from build123d import *

# Parameters (mm, degrees)
BOSS_EXTRUDE1_DEPTH = 6.35
SKETCH2_R           = 1.651
BOSS_EXTRUDE2_DEPTH = 6.35
SKETCH4_W           = 4.445
SKETCH4_H           = 4.445
BOSS_EXTRUDE3_DEPTH = 155.575


with BuildPart() as part:
    # Sketch1 → Boss-Extrude1 (new body)
    with BuildSketch(Plane.XY):
        Polygon((0, 0), (6.35, 0), (0, 14.478), (-6.35, 14.478), align=None)
    extrude(amount=BOSS_EXTRUDE1_DEPTH)

    # Sketch2 → Boss-Extrude2 (add)
    with BuildSketch(Plane.XZ):
        with BuildLine():
            Line((6.35, 18.669), (6.35, -12.319))
            ThreePointArc((6.35, -12.319), (3.175, -15.494), (0, -12.319))
            Line((0, -12.319), (0, 18.669))
            ThreePointArc((0, 18.669), (3.175, 21.844), (6.35, 18.669))
        make_face()
        with Locations((3.175, 18.669)):
            Circle(SKETCH2_R, mode=Mode.SUBTRACT)
        with Locations((3.175, -12.319)):
            Circle(SKETCH2_R, mode=Mode.SUBTRACT)
    extrude(amount=BOSS_EXTRUDE2_DEPTH)

    # Sketch4 → Boss-Extrude3 (add)
    with BuildSketch(Plane(origin=(0, 14.478, 0), x_dir=(1, 0, 0), z_dir=(0, 1, 0))):
        with Locations((-3.175, -3.175)):
            Rectangle(SKETCH4_W, SKETCH4_H)
    extrude(amount=BOSS_EXTRUDE3_DEPTH)


solid = part.part
Work out the finished part from the listing and answer in its coordinate system (mm). A direction names the side the tool comes from. Round coordinates to 2 decimals unless told otherwise and drop trailing zeros. Write each loop counter-clockwise with the first axis right and the second up, starting at its lowest first coordinate (ties: lowest second). Pieces come first, ordered by that corner, then holes. Notation, with made-up numbers: M 22,12 L 79,12 A21 ccw 79,47 Z; hole C 52.5,15 d6. An arc over 180 degrees is marked long. Use a Markdown table: item, result.
1) Consider line 1 (Z direction, x = -2.5, y = 7.5); line 2 (Z direction, x = -4.25, y = 157); line 3 (X direction, y = 74, z = 3). Determine where each line is inside the solid, lowest interval first. Write a range as [from, to].
Taken from the geometry:
| item | result |
|---|---|
| line 1 | z = [0, 6.35] |
| line 2 | z = [0.95, 5.4] |
| line 3 | x = [-5.4, -0.95] |
2) The part is cut by section B-B on y = 133. Give the vertices of the cut face in (x, z).
Taken from the geometry:
| item | result |
|---|---|
| outline | M -5.4,0.95 L -0.95,0.95 L -0.95,5.4 L -5.4,5.4 Z |
3) Flat-ended cylindrical pins translate along their axes: pin 1 (2 mm diameter, centred on x = 0, z = 11, fed in from +Y); pin 2 (5 mm diameter, centred on x = -3.5, y = 130.5, fed in from -Z); pin 3 (5 mm diameter, centred on y = 85, z = 2.5, fed in from +X). Find the tip coordinate at first contact, or state that the pin passes through.
Taken from the geometry:
| item | result |
|---|---|
| pin 1 | stops at y = 0 |
| pin 2 | stops at z = 0.95 |
| pin 3 | stops at x = -0.95 |
4) The part is cut by section C-C on z = -7.5. Give the vertices of the cut face in (x, y), plus the area to 3 significant figures.
Taken from the geometry:
| item | result |
|---|---|
| outline | M 0,-6.35 L 6.35,-6.35 L 6.35,0 L 0,0 Z |
| area | 40.3 mm2 |
5) The part is cut by section A-A on z = 3.5. Give the vertices of the cut face in (x, y).
Taken from the geometry:
| item | result |
|---|---|
| outline | M -6.35,14.48 L 0,0 L 0,-6.35 L 6.35,-6.35 L 6.35,0 L 0,14.48 L -0.95,14.48 L -0.95,170.05 L -5.4,170.05 L -5.4,14.48 Z |
6) Determine the mould class of faces 6 (the face through (3.22, 7.14, 3.13)), 7 (the face through (3.105, -3.131, 21.843)), 8 (the face through (2.96, -3.131, -10.682)), 9 (the face through (2.96, -3.131, 20.306)) for opening direction X: pulls with the +X half, pulls with the -X half, needs draft (parallel to the pull), parting line crosses it, or undercut.
Taken from the geometry:
| item | result |
|---|---|
| face 6 | pulls with the +X half |
| face 7 | parting line crosses it |
| face 8 | undercut |
| face 9 | undercut |
7) Which of the six approach directions +Z, -Z, +X, -X, +Y, -Y give full straight-line access (tool end or side, diameter ignored) to faces 1 (the face through (-3, 91, 5.398)), 2 (the face through (-5.398, 91, 3)), 3 (the face through (-0.952, 91, 3)), 4 (the face through (6.35, -3, 3)), 5 (the face through (-3, 91, 0.952))?
Taken from the geometry:
| item | result |
|---|---|
| face 1 | +Z, +X, -X, +Y |
| face 2 | +Z, -Z, -X, +Y |
| face 3 | +Z, -Z, +X, +Y |
| face 4 | +Z, -Z, +X, +Y, -Y |
| face 5 | -Z, +X, -X, +Y |
